Can you work these out from the model? Positions are in its coordinate system, mm. A direction names the side the tool comes from. Round coordinates to 2 decimals unless told otherwise and drop trailing zeros. Loops run counter-clockwise (first coordinate to the right, second up) from the corner with the lowest first, then second, coordinate; pieces in that order, holes last. Notation, with made-up numbers: M -14,76 L 12,76 A5 ccw 12,84 Z; hole C 9.5,37.25 d9. An arc over 180 degrees is marked long. Return JSON: item names as keys, results as strings.
```python
from build123d import *

# Parameters (mm, degrees)
F0_W     = 40
F0_H     = 19
F2_DEPTH = 565
F1_W     = 80
F1_H     = 100
F3_DEPTH = 25
F4_W     = 565
F4_H     = 19
F5_DEPTH = 40


with BuildPart() as f2:
    # F0 (on Right) → F2 (new body)
    with BuildSketch(Plane.YZ):
        with Locations((0, 23.5)):
            Rectangle(F0_W, F0_H)
        Polygon((20, 33), (20, 63), (17, 66), (12, 66), (12, 80), (4, 80), (4, 66), (-4, 66), (-4, 80), (-12, 80), (-12, 66), (-17, 66), (-20, 63), (-20, 33), align=None)
    extrude(amount=-F2_DEPTH)

    # F1 (on Front) → F3 (cut, symmetric)
    with BuildSketch(Plane.XZ):
        with Locations((-565, 83)):
            Rectangle(F1_W, F1_H)
    extrude(amount=F3_DEPTH, both=True, mode=Mode.SUBTRACT)

    # F4 (on face) → F5 (cut, through all)
    with BuildSketch(Plane.XZ.offset(20)):
        with Locations((-282.5, 23.5)):
            Rectangle(F4_W, F4_H)
    extrude(amount=-F5_DEPTH, mode=Mode.SUBTRACT)


solid = f2.part
```
Q1. If I drill on line 1 along Y through (x, z) = (-41, 72); line 2 along Z through (x, y) = (-55.5, 14); line 3 along Z through (x, y) = (-475, -18), over which ranges is the centre line in solid material (lowest first)?
Results:
{"line 1": "y = -12 to -4, 4 to 12", "line 2": "z = 33 to 66", "line 3": "z = 33 to 65"}
Q2. Suppose I cut it at A-A, the plane z = 74.5. Please give me the cut outline in (x, y).
Results:
{"outline": "M -525,-12 L 0,-12 L 0,-4 L -525,-4 Z; M -525,4 L 0,4 L 0,12 L -525,12 Z"}
Q3. Suppose I cut it at B-B, the plane x = -431. Please give me the cut outline in (y, z).
Results:
{"outline": "M -20,33 L 20,33 L 20,63 L 17,66 L 12,66 L 12,80 L 4,80 L 4,66 L -4,66 L -4,80 L -12,80 L -12,66 L -17,66 L -20,63 Z"}
Q4. Thinking about a two-plate mould opening in Y: for faces 4 (the flat face through (-525, 0, 51)), 5 (the flat face through (-259, 12, 73)), 6 (the flat face through (-259, 0, 66)), which applies, pulls with the +Y half, pulls with the -Y half, needs draft (parallel to the pull), parting line crosses it, or undercut?
Results:
{"face 4": "needs draft", "face 5": "pulls with the +Y half", "face 6": "undercut"}
Q5. I'm going to push flat-ended pins straight in: pin 1 Ø1 at (x, z) = (-421.5, 71) entering from +Y; pin 2 Ø7 at (x, z) = (-183, 71) entering from -Y; pin 3 Ø2.5 at (x, y) = (-297, -0.5) entering from +Z; pin 4 Ø8 at (y, z) = (16, 43.5) entering from +X. Where does each tip first touch, or does it pass through?
Results:
{"pin 1": "stops at y = 12", "pin 2": "stops at y = -12", "pin 3": "stops at z = 66", "pin 4": "stops at x = 0"}
Q6. On a 3-axis mill with a long thin cutter (end or side, diameter ignored), from which of +Z, -Z, +X, -X, +Y, -Y can I reach the whole of each face in a straight line? I mean faces 1 (the flat face through (-259, -4, 73)), 2 (the flat face through (-259, -8, 80)), 3 (the flat face through (-259, -12, 73)). Say none if no direction works.
Results:
{"face 1": "+Z, +X, -X", "face 2": "+Z, +X, -X, +Y, -Y", "face 3": "+Z, +X, -X, -Y"}
